Check sheet for the drawn part. Datum: minimum x, y, z corner. Units: mm. A direction names the side the tool comes from. Give positions to 0.01 mm unless a question says otherwise; leave off trailing zeros. Order: outer loops, then holes, each group sorted by start corner. A loop starts at its lowest first (then second) coordinate and runs counter-clockwise, first axis right, second up. Notation, with made-up numbers: (3, -29) - (32, -29) arc R27 ccw to (32, 7) - close; hole circle Ø11 at (-29.75, -23). An arc over 180 degrees is marked (long way). Answer as a JSON object with one key per item and string values. Group by question number.
(1) Section check A-A (x = 15). Record the boundary of the cut face in (y, z).
(2) Depth check by flat-ended pin: pin 1 Ø1.5 at (y, z) = (18.5, 15.5) entering from +X; pin 2 Ø6 at (x, y) = (8.5, 15.5) entering from +Z. Enter the tip coordinate at first touch or a pass-through.
(3) Access from +Z, -Z, +X, -X, +Y, -Y to the whole of each face (thin tool, end or side, straight path). Record for the marked faces 1 and 2.
(4) Mould release check, pull along Y, two halves, no side actions. Record for the marked faces 3, 4, 5 and 6: +Y half, -Y half, draft (parallel to the pull), parting line (faces both ways), or undercut.
(5) Section check D-D (y = 20.75). Record the boundary of the cut face in (x, z).
(6) Section check B-B (y = 15.25). Record the boundary of the cut face in (x, z).
(7) Section check C-C (x = 3.25). Record the boundary of the cut face in (y, z) (1 decimal).
(8) Thickness scan on line 1 (Z direction, x = 8.25, y = 9.25); line 2 (X direction, y = 9, z = 7.25); line 3 (X direction, y = 17.25, z = 4.75) (1 decimal). Record the ranges inside material, lowest first.
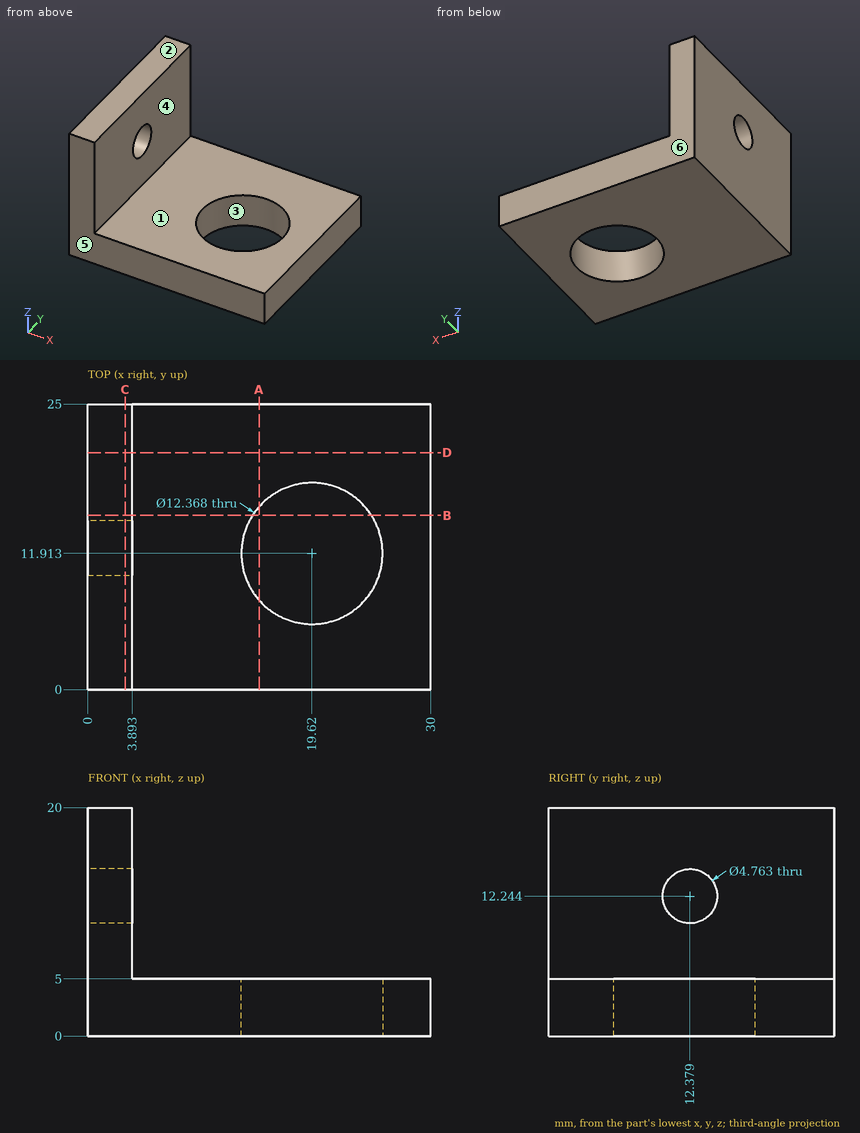
Solutions:
{
 "1": {"outline": "(0, 0) - (7.8, 0) - (7.8, 5) - (0, 5) - close; (16.02, 0) - (25, 0) - (25, 5) - (16.02, 5) - close"},
 "2": {"pin 1": "stops at x = 3.89", "pin 2": "stops at z = 5"},
 "3": {"face 1": "+Z, +X, +Y, -Y", "face 2": "+Z, +X, -X, +Y, -Y"},
 "4": {"face 3": "undercut", "face 4": "draft", "face 5": "-Y half", "face 6": "+Y half"},
 "5": {"outline": "(0, 0) - (30, 0) - (30, 5) - (3.89, 5) - (3.89, 20) - (0, 20) - close"},
 "6": {"outline": "(0, 0) - (14.41, 0) - (14.41, 5) - (3.89, 5) - (3.89, 20) - (0, 20) - close; (24.83, 0) - (30, 0) - (30, 5) - (24.83, 5) - close"},
 "7": {"outline": "(0, 0) - (25, 0) - (25, 20) - (0, 20) - close; hole circle Ø4.8 at (12.4, 12.2)"},
 "8": {"line 1": "z = 0 to 5", "line 2": "x = 0 to 3.89", "line 3": "x = 0 to 16.5, 22.7 to 30"}
}
